```python
from build123d import *

# Parameters (mm, degrees)
SKETCH1_W                                           = 1.6
SKETCH1_H                                           = 3.5
CBORE_FOR_M3_HEX_SOCKET_HEAD_CAP_SCREW2_D           = 3.4
CBORE_FOR_M3_HEX_SOCKET_HEAD_CAP_SCREW2_DEPTH       = 8.566
CBORE_FOR_M3_HEX_SOCKET_HEAD_CAP_SCREW2_CBORE_D     = 6.5
CBORE_FOR_M3_HEX_SOCKET_HEAD_CAP_SCREW2_CBORE_DEPTH = 3.4
CBORE_FOR_M3_HEX_SOCKET_HEAD_CAP_SCREW2_TIP         = 1.021463052
CHAMFER1_SIZE                                       = 1


with BuildPart() as part:
    # Sketch1 → Revolve17 (revolve)
    with BuildSketch(Plane.XY, mode=Mode.PRIVATE) as revolve17_sk:
        Polygon((-13.572880732, 3.15), (-13.572880732, 3.85), (-17.906214066, 3.15), (-17.906214066, 1.9), (0, 1.9), (14.469928658, 18.9), (15.469928658, 18.9), (15.469928658, 22.4), (15.469928658, 24.5), (16.469928658, 24.5), (16.469928658, 35), (7.903928658, 35), (7.903928658, 18.9), (-4.906214066, 3.85), (-9.239547399, 3.15), (-9.239547399, 3.85), align=None)
        with Locations((16.269928658, 20.65)):
            Rectangle(SKETCH1_W, SKETCH1_H)
    revolve(revolve17_sk.sketch.rotate(Axis((-801.920554309, 0, 0), (1, 0, 0)), 90), axis=Axis((-801.920554309, 0, 0), (1, 0, 0)))

    # CBORE for M3 Hex Socket Head Cap Screw2
    with Locations(Plane.ZY.offset(-7.903928658)):
        with Locations((-21.001071401, -21.154915542), (0, 29.7), (29.7, 0), (-29.7, 0), (0, -29.7), (-21.001071401, 20.847227261), (21.001071401, 20.847227261), (21.001071401, -21.154915542)):
            CounterBoreHole(CBORE_FOR_M3_HEX_SOCKET_HEAD_CAP_SCREW2_D / 2, CBORE_FOR_M3_HEX_SOCKET_HEAD_CAP_SCREW2_CBORE_D / 2, CBORE_FOR_M3_HEX_SOCKET_HEAD_CAP_SCREW2_CBORE_DEPTH, depth=CBORE_FOR_M3_HEX_SOCKET_HEAD_CAP_SCREW2_DEPTH)
            with Locations((0, 0, -(CBORE_FOR_M3_HEX_SOCKET_HEAD_CAP_SCREW2_DEPTH + CBORE_FOR_M3_HEX_SOCKET_HEAD_CAP_SCREW2_TIP / 2))):  # 118° drill point
                Cone(0, CBORE_FOR_M3_HEX_SOCKET_HEAD_CAP_SCREW2_D / 2, CBORE_FOR_M3_HEX_SOCKET_HEAD_CAP_SCREW2_TIP, mode=Mode.SUBTRACT)

    # Chamfer1
    chamfer1_edges = [part.edges().sort_by_distance(p)[0] for p in [
        (7.903928658, 0, -35),
    ]]
    chamfer(chamfer1_edges, length=CHAMFER1_SIZE)


solid = part.part
```
Input: part model. Units: mm. Frame: model coordinates. A direction names the side the tool comes from. Round coordinates to 2 decimals unless told otherwise and drop trailing zeros. Loops run counter-clockwise (first coordinate to the right, second up) from the corner with the lowest first, then second, coordinate; pieces in that order, holes last. Notation, with made-up numbers: (66, 9) -> (90, 9) arc R26 ccw to (90, 43) -> close; hole circle Ø4 at (-34.5, -0.5). An arc over 180 degrees is marked (long way). One line per item, written item: value.
(1) Section D-D (x = -6). Return the cut outline in (y, z).
Geometry check:
outline: circle Ø7.35 at (0, 0); hole circle Ø3.8 at (0, 0)
(2) Mould query, pull axis X, two halves, no side actions, for faces 1 (the face through (-8.828, -0.571, 1.812)), 2 (the face through (7.904, 15, 15)), 3 (the face through (17.07, 15, 12)), 4 (the face through (-7.58, 3.03, 1.58)). Classes: pulls with the +X half, pulls with the -X half, needs draft (parallel to the pull), parting line crosses it, or undercut.
Geometry check:
face 1: needs draft
face 2: pulls with the -X half
face 3: pulls with the +X half
face 4: undercut
(3) Pin query (flat end, axial travel): pin 1 (6 mm diameter, centred on x = 11.5, z = 9, fed in from -Y); pin 2 (1.5 mm diameter, centred on x = 5.5, y = 9.5, fed in from -Z); pin 3 (4 mm diameter, centred on y = 0, z = 29.7, fed in from +X). Return the tip coordinate at first contact, or that it passes through.
Geometry check:
pin 1: y = -34.48
pin 2: z = -14.16
pin 3: x = 16.47
(4) Material intervals for line 1 (Y direction, x = 16.05, z = 0); line 2 (Z direction, x = 13.5, y = 22); line 3 (Y direction, x = 13.5, z = 31), sorted ascending. Write a range as [from, to].
Geometry check:
line 1: [-35, -31.4], [-28, -24.5], [-22.4, -18.9], [18.9, 22.4], [24.5, 28], [31.4, 35]
line 2: [-27.22, -22.25], [-19.75, 19.75], [22.25, 27.22]
line 3: [-16.25, -1.1], [1.1, 16.25]
(5) Section A-A (x = 12.5). Give the number of separate pieces and of enclosed holes in the cut face, plus the area to 3 significant figures.
Geometry check:
separate pieces: 1
enclosed holes: 9
area: 2,910 mm2
(6) Set-up query: faces 5 (the face through (13.92, 0.51, 28.08)), 6 (the face through (15.47, 11, -20)), 7 (the face through (11.304, 19, -20)). Return all of +Z, -Z, +X, -X, +Y, -Y with unobstructed straight access to the full face (end or side cutting, diameter ignored); none if empty.
Geometry check:
face 5: +X, -X
face 6: +X
face 7: -X
